```python
from build123d import *

# Parameters (mm, degrees)
PAD_DEPTH       = 60
SKETCH001_W     = 30
SKETCH001_H     = 45
POCKET_DEPTH    = 5
SKETCH002_R     = 1.75
POCKET001_DEPTH = 5.001
CHAMFER_SIZE    = 1.2
CHAMFER001_SIZE = 0.6
CHAMFER002_SIZE = 0.4


with BuildPart() as part:
    # Sketch → Pad (new body)
    with BuildSketch(Plane.YZ):
        with BuildLine():
            Line((-45, -4), (-45, 0))
            Line((-45, 0), (0, 0))
            Line((0, 0), (0, 30))
            Line((0, 30), (5, 30))
            Line((5, 30), (5.283101, 30))
            ThreePointArc((5.283101, 30), (11.950524, 7.386027), (33.4, -2.4))
            Line((33.4, -2.4), (33.4, -4))
            Line((33.4, -4), (0, -4))
            Line((0, -4), (-33.175, -4))
            Line((-33.175, -4), (-33.175, -5))
            Line((-33.175, -5), (-38.65, -5))
            Line((-38.65, -5), (-38.65, -4))
            Line((-38.65, -4), (-45, -4))
        make_face()
    extrude(amount=PAD_DEPTH)

    # Sketch001 → Pocket (cut)
    with BuildSketch(Plane.XY):
        with Locations((15, -22.5)):
            Rectangle(SKETCH001_W, SKETCH001_H)
    extrude(amount=-POCKET_DEPTH, mode=Mode.SUBTRACT)

    # Sketch002 → Pocket001 (cut, through all)
    with BuildSketch(Plane.XY):
        with Locations((45, -35.9125)):
            Circle(SKETCH002_R)
    extrude(amount=-POCKET001_DEPTH, mode=Mode.SUBTRACT)

    # Chamfer
    chamfer_edges = [part.edges().sort_by_distance(p)[0] for p in [
        (30, 0, -2),
        (45, 0, 0),
        (60, -45, -2),
        (30, -45, -2),
    ]]
    chamfer(chamfer_edges, length=CHAMFER_SIZE)

    # Chamfer001
    chamfer001_edges = [part.edges().sort_by_distance(p)[0] for p in [
        (43.25, -35.9125, 0),
    ]]
    chamfer(chamfer001_edges, length=CHAMFER001_SIZE)

    # Chamfer002
    chamfer002_edges = [part.edges().sort_by_distance(p)[0] for p in [
        (60, -22.5, 0),
        (60, -43.8, -2),
        (60, -0.6, 0.6),
        (60, -41.225, -4),
        (60, 0, 15.6),
        (60, -38.65, -4.5),
        (60, 2.641551, 30),
        (60, -35.9125, -5),
        (60, 11.950524, 7.386027),
        (60, -33.175, -4.5),
        (60, 33.4, -3.2),
        (60, 0.1125, -4),
    ]]
    chamfer(chamfer002_edges, length=CHAMFER002_SIZE)


solid = part.part
```
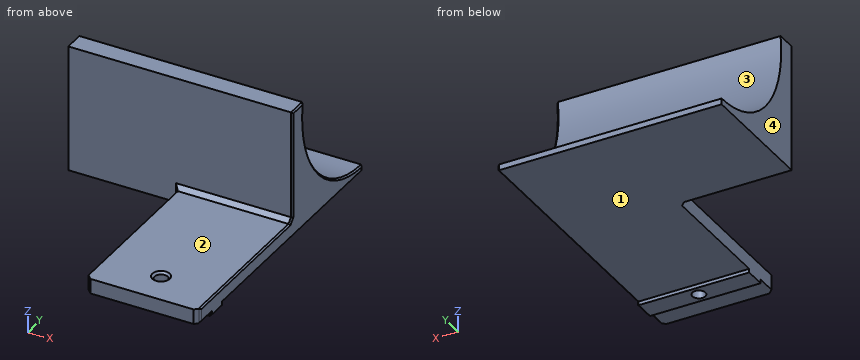
Check sheet for the modelled part. Datum: model origin and axes. Units: mm. Face numbers are marked on the shaded views. Round coordinates to 2 decimals unless told otherwise and drop trailing zeros. Order: outer loops, then holes, each group sorted by start corner. A loop starts at its lowest first (then second) coordinate and runs counter-clockwise, first axis right, second up. Notation, with made-up numbers: (3, 83.25) - (57, 83.25) arc R22 ccw to (57, 116.25) - close; hole circle Ø10 at (28.25, 37). An arc over 180 degrees is marked (long way). Answer as CSV lines item,"result". Start each with the question number.
1) Section check B-B (x = 36.5). Record the cut outline in (y, z) (3 decimals), then the cut area to 3 significant figures.
2) Section check C-C (y = -4). Record the cut outline in (x, z), then the cut area to 3 significant figures.
3) Section check D-D (x = 27). Record the cut outline in (y, z).
4) Scan lines: probe 1 along Y at (x, z) = (45, -3); probe 2 along Y at (x, z) = (34, 27); probe 3 along Z at (x, y) = (46, -9). Record each from-to range of solid material in increasing order.
5) Depth check by flat-ended pin: pin 1 (0.8 mm diameter, centred on x = 38.5, z = -4.5, fed in from -Y); pin 2 (6 mm diameter, centred on x = 46.5, y = 22.5, fed in from +Z); pin 3 (2 mm diameter, centred on x = 34, z = 14, fed in from +Y). Enter the tip coordinate at first touch or a pass-through.
6) Draft check along Z on the marked faces 1, 2, 3 and 4. Enter one of: +Z half, -Z half, draft (parallel to the pull), parting line (faces both ways), or undercut.
Determined:
1,outline,"(-45, -4) - (-38.65, -4) - (-38.65, -5) - (-33.175, -5) - (-33.175, -4) - (33.4, -4) - (33.4, -2.4) arc R28.4 cw to (5.283, 30) - (0, 30) - (0, 1.2) - (-1.2, 0) - (-45, 0) - close"
1,area,"575 mm^2"
2,outline,"(30, -4) - (59.6, -4) - (60, -3.6) - (60, -0.4) - (59.6, 0) - (30, 0) - close"
2,area,"120 mm^2"
3,outline,"(0, -4) - (33.4, -4) - (33.4, -2.4) arc R28.4 cw to (5.28, 30) - (0, 30) - close"
4,probe 1,"-45 to -37.66, -34.16 to 33.4"
4,probe 2,"0 to 5.02"
4,probe 3,"-4 to 0"
5,pin 1,"y = -38.65"
5,pin 2,"z = 1.23"
5,pin 3,"y = 8.15"
6,face 1,"-Z half"
6,face 2,"+Z half"
6,face 3,"undercut"
6,face 4,"draft"
